```python
from build123d import *

# Parameters (mm, degrees)
SKETCH1_W                    = 2220
SKETCH1_H                    = 969
BASE_FLANGE1_DEPTH           = 4
EDGE_FLANGE1_START           = -788.522727273
EDGE_FLANGE1_DEPTH           = 2220
EDGE_FLANGE1_2_DEPTH         = 2220
EDGE_FLANGE2_START           = -788.522727273
EDGE_FLANGE2_DEPTH           = 2220
EDGE_FLANGE2_2_DEPTH         = 2220
EDGE_FLANGE3_STRIP_W         = 24
EDGE_FLANGE3_STRIP_H         = 4
EDGE_FLANGE3_STRIP_CUT_DEPTH = 954.890119211
EDGE_FLANGE3_DEPTH           = 954.890119211
EDGE_FLANGE4_STRIP_W         = 24
EDGE_FLANGE4_STRIP_H         = 4
EDGE_FLANGE4_STRIP_CUT_DEPTH = 954.890119211
EDGE_FLANGE4_DEPTH           = 954.890119211
CUT_EXTRUDE1_DEPTH           = 1665.596730593
LPATTERN1_COUNT              = 7
LPATTERN1_PITCH              = 300
CUT_EXTRUDE2_DEPTH           = 1665.596730593
CUT_EXTRUDE2_DEPTH_BACK      = 1665.596730593
SKETCH20_R                   = 7
CUT_EXTRUDE3_DEPTH           = 2327.247497544
LPATTERN2_COUNT              = 5
LPATTERN2_PITCH              = 190
CUT_EXTRUDE4_DEPTH           = 1704.160586281
LPATTERN3_COUNT              = 7
LPATTERN3_PITCH              = 300
CUT_EXTRUDE5_DEPTH           = 1704.160586281
CUT_EXTRUDE5_DEPTH_BACK      = 1704.160586281


# Read off the part's stored shape, not the designer's step: Edge-Flange1, Edge-Flange2
# Sheet-metal steps are written as plain solids
with BuildPart() as part:
    # Sketch1 → Base-Flange1 (new body)
    with BuildSketch(Plane(origin=(0, 0, 0), x_dir=(0, 0, -1), z_dir=(1, 0, 0))):
        with Locations((-321.477272727, 132.136363636)):
            Rectangle(SKETCH1_W, SKETCH1_H)
    extrude(amount=-BASE_FLANGE1_DEPTH)

    # Edge-Flange1 outline → Edge-Flange1 (cut)
    with BuildSketch(Plane.XY.offset(EDGE_FLANGE1_START)):
        with BuildLine():
            ThreePointArc((-4, 609.581423242), (-3.220682275, 613.025512017), (-1.034563128, 615.798590934))
            Line((-1.034563128, 615.798590934), (0, 616.636363636))
            Line((0, 616.636363636), (-4, 616.636363636))
            Line((-4, 616.636363636), (-4, 609.581423242))
        make_face()
    extrude(amount=EDGE_FLANGE1_DEPTH, mode=Mode.SUBTRACT)

    # Edge-Flange1 2 outline → Edge-Flange1 2 (add)
    with BuildSketch(Plane.XY.offset(EDGE_FLANGE1_START)):
        with BuildLine():
            Line((89.257515375, 688.91567443), (0, 616.636363636))
            Line((0, 616.636363636), (0, 609.581423242))
            ThreePointArc((0, 609.581423242), (0.389658863, 611.303467629), (1.482718436, 612.690007088))
            Line((1.482718436, 612.690007088), (91.774796939, 685.807090584))
            Line((91.774796939, 685.807090584), (89.257515375, 688.91567443))
        make_face()
    extrude(amount=EDGE_FLANGE1_2_DEPTH)

    # Edge-Flange2 outline → Edge-Flange2 (cut)
    with BuildSketch(Plane.XY.offset(EDGE_FLANGE2_START)):
        with BuildLine():
            ThreePointArc((0, -345.308695969), (-0.779317725, -348.752784744), (-2.965436872, -351.525863661))
            Line((-2.965436872, -351.525863661), (-4, -352.363636364))
            Line((-4, -352.363636364), (0, -352.363636364))
            Line((0, -352.363636364), (0, -345.308695969))
        make_face()
    extrude(amount=EDGE_FLANGE2_DEPTH, mode=Mode.SUBTRACT)

    # Edge-Flange2 2 outline → Edge-Flange2 2 (add)
    with BuildSketch(Plane.XY.offset(EDGE_FLANGE2_START)):
        with BuildLine():
            Line((-38.857298073, -380.590519783), (-4, -352.363636364))
            Line((-4, -352.363636364), (-4, -345.308695969))
            ThreePointArc((-4, -345.308695969), (-4.389658863, -347.030740356), (-5.482718436, -348.417279815))
            Line((-5.482718436, -348.417279815), (-41.374579637, -377.481935938))
            Line((-41.374579637, -377.481935938), (-38.857298073, -380.590519783))
        make_face()
    extrude(amount=EDGE_FLANGE2_2_DEPTH)

    # Edge-Flange3 strip (across the edge) → Edge-Flange3 strip cut (cut)
    with BuildSketch(Plane(origin=(-4, -345.308695969, 1431.477272727), x_dir=(0, 0, -1), z_dir=(0, 1, 0))):
        with Locations((-4, -2)):
            Rectangle(EDGE_FLANGE3_STRIP_W, EDGE_FLANGE3_STRIP_H)
    extrude(amount=EDGE_FLANGE3_STRIP_CUT_DEPTH, mode=Mode.SUBTRACT)

    # Edge-Flange3 section (across the edge) → Edge-Flange3 (add)
    with BuildSketch(Plane(origin=(-4, -345.308695969, 1431.477272727), x_dir=(0, 0, -1), z_dir=(0, 1, 0))):
        with BuildLine():
            Line((0, 4), (0, 46))
            Line((0, 46), (4, 46))
            Line((4, 46), (4, 4))
            ThreePointArc((4, 4), (5.171572875, 1.171572875), (8, 0))
            Line((8, 0), (8, -4))
            ThreePointArc((8, -4), (2.343145751, -1.656854249), (0, 4))
        make_face()
    extrude(amount=EDGE_FLANGE3_DEPTH)

    # Edge-Flange4 strip (across the edge) → Edge-Flange4 strip cut (cut)
    with BuildSketch(Plane(origin=(-4, 609.581423242, -788.522727273), x_dir=(0, 0, 1), z_dir=(0, -1, 0))):
        with Locations((-4, -2)):
            Rectangle(EDGE_FLANGE4_STRIP_W, EDGE_FLANGE4_STRIP_H)
    extrude(amount=EDGE_FLANGE4_STRIP_CUT_DEPTH, mode=Mode.SUBTRACT)

    # Edge-Flange4 section (across the edge) → Edge-Flange4 (add)
    with BuildSketch(Plane(origin=(-4, 609.581423242, -788.522727273), x_dir=(0, 0, 1), z_dir=(0, -1, 0))):
        with BuildLine():
            Line((0, 4), (0, 46))
            Line((0, 46), (4, 46))
            Line((4, 46), (4, 4))
            ThreePointArc((4, 4), (5.171572875, 1.171572875), (8, 0))
            Line((8, 0), (8, -4))
            ThreePointArc((8, -4), (2.343145751, -1.656854249), (0, 4))
        make_face()
    extrude(amount=EDGE_FLANGE4_DEPTH)

    # Sketch18 → Cut-Extrude1 (cut, symmetric)
    with BuildSketch(Plane(origin=(-301.580689808, 372.42113631, 0), x_dir=(0.7771459614569678, 0.6293203910498413, 0), z_dir=(-0.6293203910498413, 0.7771459614569678, 0))):
        with BuildLine():
            Line((484.914799236, 643.522727273), (484.914799236, 633.522727273))
            ThreePointArc((484.914799236, 633.522727273), (477.914799236, 626.522727273), (470.914799236, 633.522727273))
            Line((470.914799236, 633.522727273), (470.914799236, 643.522727273))
            ThreePointArc((470.914799236, 643.522727273), (477.914799236, 650.522727273), (484.914799236, 643.522727273))
        make_face()
    cut_extrude1 = extrude(amount=CUT_EXTRUDE1_DEPTH, both=True, mode=Mode.SUBTRACT)

    # LPattern1: Cut-Extrude1 ×7
    with Locations(*[(0, 0, i * LPATTERN1_PITCH) for i in range(1, LPATTERN1_COUNT)]):
        add(cut_extrude1, mode=Mode.SUBTRACT)

    # Sketch19 → Cut-Extrude2 (cut, two sides: drawn at the far end of the back side and taken through both)
    with BuildSketch(Plane(origin=(-301.580689808, 372.42113631, 0), x_dir=(0.7771459614569678, 0.6293203910498413, 0), z_dir=(-0.6293203910498413, 0.7771459614569678, 0)).offset(-CUT_EXTRUDE2_DEPTH_BACK)):
        with BuildLine():
            Line((484.914799236, -1336.477272727), (484.914799236, -1346.477272727))
            ThreePointArc((484.914799236, -1346.477272727), (477.914799236, -1353.477272727), (470.914799236, -1346.477272727))
            Line((470.914799236, -1346.477272727), (470.914799236, -1336.477272727))
            ThreePointArc((470.914799236, -1336.477272727), (477.914799236, -1329.477272727), (484.914799236, -1336.477272727))
        make_face()
    extrude(amount=CUT_EXTRUDE2_DEPTH + CUT_EXTRUDE2_DEPTH_BACK, mode=Mode.SUBTRACT)

    # Sketch20 → Cut-Extrude3 (cut, symmetric)
    with BuildSketch(Plane.XY.offset(1431.477272727)):
        with Locations((-25, -246.525863661)):
            Circle(SKETCH20_R)
    cut_extrude3 = extrude(amount=CUT_EXTRUDE3_DEPTH, both=True, mode=Mode.SUBTRACT)

    # LPattern2: Cut-Extrude3 ×5
    with Locations(*[(0, i * LPATTERN2_PITCH, 0) for i in range(1, LPATTERN2_COUNT)]):
        add(cut_extrude3, mode=Mode.SUBTRACT)

    # Sketch21 → Cut-Extrude4 (cut, symmetric)
    with BuildSketch(Plane(origin=(168.230364565, -207.747198844, 0), x_dir=(0.7771459614569676, 0.6293203910498416, 0), z_dir=(-0.6293203910498416, 0.7771459614569677, 0))):
        with BuildLine():
            Line((-237.71116701, 643.522727273), (-237.71116701, 633.522727273))
            ThreePointArc((-237.71116701, 633.522727273), (-244.71116701, 626.522727273), (-251.71116701, 633.522727273))
            Line((-251.71116701, 633.522727273), (-251.71116701, 643.522727273))
            ThreePointArc((-251.71116701, 643.522727273), (-244.71116701, 650.522727273), (-237.71116701, 643.522727273))
        make_face()
    cut_extrude4 = extrude(amount=CUT_EXTRUDE4_DEPTH, both=True, mode=Mode.SUBTRACT)

    # LPattern3: Cut-Extrude4 ×7
    with Locations(*[(0, 0, i * LPATTERN3_PITCH) for i in range(1, LPATTERN3_COUNT)]):
        add(cut_extrude4, mode=Mode.SUBTRACT)

    # Sketch22 → Cut-Extrude5 (cut, two sides: drawn at the far end of the back side and taken through both)
    with BuildSketch(Plane(origin=(168.230364565, -207.747198844, 0), x_dir=(0.7771459614569676, 0.6293203910498416, 0), z_dir=(-0.6293203910498416, 0.7771459614569677, 0)).offset(-CUT_EXTRUDE5_DEPTH_BACK)):
        with BuildLine():
            Line((-237.71116701, -1356.477272727), (-237.71116701, -1366.477272727))
            ThreePointArc((-237.71116701, -1366.477272727), (-244.71116701, -1373.477272727), (-251.71116701, -1366.477272727))
            Line((-251.71116701, -1366.477272727), (-251.71116701, -1356.477272727))
            ThreePointArc((-251.71116701, -1356.477272727), (-244.71116701, -1349.477272727), (-237.71116701, -1356.477272727))
        make_face()
    extrude(amount=CUT_EXTRUDE5_DEPTH + CUT_EXTRUDE5_DEPTH_BACK, mode=Mode.SUBTRACT)


solid = part.part
```
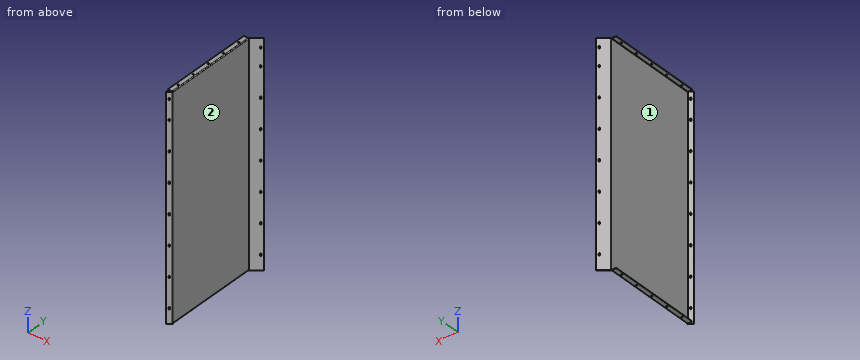
Work out the finished part from the listing and answer in its coordinate system (mm). Face numbers are marked on the shaded views. Coordinates: 2 decimals unless noted, no trailing zeros. Write each loop counter-clockwise with the first axis right and the second up, starting at its lowest first coordinate (ties: lowest second). Pieces come first, ordered by that corner, then holes.
Q1. Each of these flat-tipped pins is pushed along its axis until it touches: pin 1 Ø8 at (y, z) = (250.5, -211) entering from +X; pin 2 Ø1.2 at (x, z) = (-2, 1429) entering from +Y; pin 3 Ø2 at (x, z) = (-2, -784) entering from +Y. Where does it stop, or does it pass through?
Q2. A cutting plane is placed at C-C, the plane x = 32. Give the vertices of the cut face in (y, z).
Q3. A cutting plane is placed at B-B, the plane z = -75. Give the vertices of the cut face in (x, y).
Q4. A cutting plane is placed at A-A, the plane y = 266. Give the vertices of the cut face in (x, z), then the cut area to 3 significant figures.
Q5. Find the intervals of material crossed by line 1 (Z direction, x = -21, y = -6.5); line 2 (X direction, y = 34.5, z = 697.5); line 3 (Y direction, x = -13, z = -40), in increasing order.
Q6. Determine the mould class of the marked faces 1 and 2 for opening direction Z: released by +Z, released by -Z, zero draft, split by the parting line, or undercut.
Findings below:
1. pin 1: stops at x = 0
1. pin 2: stops at y = 615.48
1. pin 3: stops at y = 615.83
2. outline: (637.4, -788.52) - (642.55, -788.52) - (642.55, 1431.48) - (637.4, 1431.48) - close
3. outline: (-41.37, -377.48) - (-38.86, -380.59) - (-2.97, -351.53) arc R8 ccw to (0, -345.31) - (0, 609.58) arc R4 cw to (1.48, 612.69) - (91.77, 685.81) - (89.26, 688.92) - (-1.03, 615.8) arc R8 ccw to (-4, 609.58) - (-4, -345.31) arc R4 cw to (-5.48, -348.42) - close
4. outline: (-50, -788.52) - (-8, -788.52) arc R8 ccw to (0, -780.52) - (0, 1423.48) arc R8 ccw to (-8, 1431.48) - (-50, 1431.48) - (-50, 1427.48) - (-8, 1427.48) arc R4 cw to (-4, 1423.48) - (-4, -780.52) arc R4 cw to (-8, -784.52) - (-50, -784.52) - close
4. area: 9,230 mm2
5. line 1: z = -788.52 to -784.52, 1427.48 to 1431.48
5. line 2: x = -4 to 0
5. line 3: y = -359.65 to -354.5
6. face 1: undercut
6. face 2: zero draft
